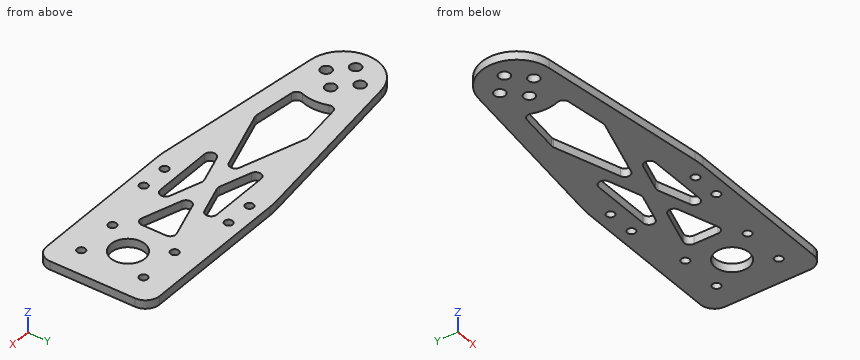
```python
from build123d import *

# Parameters (mm, degrees)
EXTRUDE_1_DEPTH          = 3
CUT_EXTRUDE_1_DEPTH      = 123.185310083
CUT_EXTRUDE_1_DEPTH_BACK = 123.185310083
SKETCH_2_R               = 1.95
FILLET_1_R               = 5
SKETCH_3_R               = 1.45
CUT_EXTRUDE_2_DEPTH      = 123.185310083
SKETCH_4_R               = 1.45
CUT_EXTRUDE_3_DEPTH      = 123.185310083
FILLET_2_R               = 30
SKETCH_6_R               = 6
CUT_EXTRUDE_4_DEPTH      = 123.185310083
FILLET_3_R               = 2


with BuildPart() as part:
    # 草图1 → 凸台-拉伸1 (new body)
    with BuildSketch(Plane.XY):
        with BuildLine():
            Line((60.5, 20), (120.5, 20))
            Line((120.5, 20), (120.5, -20))
            Line((120.5, -20), (60.5, -20))
            Line((60.5, -20), (-1.51896419, -12.407366674))
            ThreePointArc((-1.51896419, -12.407366674), (-12.5, 0), (-1.51896419, 12.407366674))
            Line((-1.51896419, 12.407366674), (60.5, 20))
        make_face()
    extrude(amount=EXTRUDE_1_DEPTH)

    # 草图2 → 切除-拉伸1 (cut, two sides: drawn at the far end of the back side and taken through both)
    with BuildSketch(Plane.XY.offset(3).offset(-CUT_EXTRUDE_1_DEPTH_BACK)):
        with Locations((0, 6)):
            Circle(SKETCH_2_R)
        with Locations((6, 0)):
            Circle(SKETCH_2_R)
        with Locations((0, -6)):
            Circle(SKETCH_2_R)
        with Locations((-6, 0)):
            Circle(SKETCH_2_R)
    extrude(amount=CUT_EXTRUDE_1_DEPTH + CUT_EXTRUDE_1_DEPTH_BACK, mode=Mode.SUBTRACT)

    # 圆角1
    fillet_1_edges = [part.edges().sort_by_distance(p)[0] for p in [
        (120.5, 20, 1.5),
        (120.5, -20, 1.5),
    ]]
    fillet(fillet_1_edges, radius=FILLET_1_R)

    # 草图3 → 切除-拉伸2 (cut, through all)
    with BuildSketch(Plane(origin=(0, 0, 0), x_dir=(-1, 0, 0), z_dir=(0, 0, -1))):
        with Locations((-111, -11)):
            Circle(SKETCH_3_R)
        with Locations((-111, 11)):
            Circle(SKETCH_3_R)
        with Locations((-96, 11)):
            Circle(SKETCH_3_R)
        with Locations((-96, -11)):
            Circle(SKETCH_3_R)
    extrude(amount=-CUT_EXTRUDE_2_DEPTH, mode=Mode.SUBTRACT)

    # 草图4 → 切除-拉伸3 (cut, through all)
    with BuildSketch(Plane.XY.offset(3)):
        with Locations((75.5, 15)):
            Circle(SKETCH_4_R)
        with Locations((65.5, 15)):
            Circle(SKETCH_4_R)
        with Locations(Location((65.5, -15, 0), (0, 0, 180))):
            Circle(SKETCH_4_R)
        with Locations(Location((75.5, -15, 0), (0, 0, 180))):
            Circle(SKETCH_4_R)
    extrude(amount=-CUT_EXTRUDE_3_DEPTH, mode=Mode.SUBTRACT)

    # 圆角2
    fillet_2_edges = [part.edges().sort_by_distance(p)[0] for p in [
        (60.5, 20, 1.5),
        (60.5, -20, 1.5),
    ]]
    fillet(fillet_2_edges, radius=FILLET_2_R)

    # 草图6 → 切除-拉伸4 (cut, through all)
    with BuildSketch(Plane.XY.offset(3)):
        with Locations((103.5, 0)):
            Circle(SKETCH_6_R)
        with BuildLine():
            Line((12.110641117, 7.023700714), (29.621886423, 9.167504088))
            Line((29.621886423, 9.167504088), (58.382978877, 0))
            Line((58.382978877, 0), (29.621886423, -9.167504088))
            Line((29.621886423, -9.167504088), (12.110641117, -7.023700714))
            ThreePointArc((12.110641117, -7.023700714), (14, 0), (12.110641117, 7.023700714))
        make_face()
        Polygon((40.181331173, -10), (63.710984536, -2.5), (87.240637899, -10), align=None)
        Polygon((40.181331173, 10), (63.710984536, 2.5), (87.240637899, 10), align=None)
        Polygon((91, 7), (69.038990194, 0), (91, -7), align=None)
    extrude(amount=-CUT_EXTRUDE_4_DEPTH, mode=Mode.SUBTRACT)

    # 圆角3
    fillet_3_edges = [part.edges().sort_by_distance(p)[0] for p in [
        (40.181331173, 10, 1.5),
        (87.240637899, 10, 1.5),
        (63.710984536, 2.5, 1.5),
        (91, 7, 1.5),
        (91, -7, 1.5),
        (69.038990194, 0, 1.5),
        (87.240637899, -10, 1.5),
        (40.181331173, -10, 1.5),
        (63.710984536, -2.5, 1.5),
        (12.110641117, -7.023700714, 1.5),
        (12.110641117, 7.023700714, 1.5),
        (29.621886423, 9.167504088, 1.5),
        (58.382978877, 0, 1.5),
        (29.621886423, -9.167504088, 1.5),
    ]]
    fillet(fillet_3_edges, radius=FILLET_3_R)


solid = part.part
```
Geometry check sheet. Reference: the model listing, model coordinates, mm. Round coordinates to 2 decimals unless told otherwise and drop trailing zeros. Order: outer loops, then holes, each group sorted by start corner. A loop starts at its lowest first (then second) coordinate and runs counter-clockwise, first axis right, second up. Notation, with made-up numbers: (57.5, -6.75) - (100.5, -6.75) arc R27 cw to (100.5, 19.25) - close; hole circle Ø7 at (10.25, 45). An arc over 180 degrees is marked (long way). Use a Markdown table: item, result. Add a question column.
(1) Sectioned sample at D-D, the plane x = 37. Enter the section's corners in (y, z).
(2) Material ranges on line 1 along Y through (x, z) = (111, 1.85); line 2 along Y through (x, z) = (71.5, 2.35); line 3 along Y through (x, z) = (103.5, 0.75), recorded low to high. Write a range as [from, to].
(3) Depth check by flat-ended pin: pin 1 (1 mm diameter, centred on y = 7.5, z = 0.5, fed in from -X). Enter the tip coordinate at first touch or a pass-through.
(4) Sectioned sample at B-B, the plane x = 65.5. Enter the section's corners in (y, z).
(5) Sectioned sample at A-A, the plane x = 103.5. Enter the section's corners in (y, z).
(6) Sectioned sample at C-C, the plane z = 0.85. Count the separate pieces of the cut face and the enclosed holes in it, and give its area (3 significant figures).
Answers below:
| question | item | result |
|---|---|---|
| 1 | outline | (-17.12, 0) - (-6.82, 0) - (-6.82, 3) - (-17.12, 3) - close; (6.82, 0) - (17.12, 0) - (17.12, 3) - (6.82, 3) - close |
| 2 | line 1 | [-20, -12.45], [-9.55, 9.55], [12.45, 20] |
| 2 | line 2 | [-20, -10], [-4.98, 4.98], [10, 20] |
| 2 | line 3 | [-20, -6], [6, 20] |
| 3 | pin 1 | x = -10.36 |
| 4 | outline | (-20, 0) - (-16.45, 0) - (-16.45, 3) - (-20, 3) - close; (-13.55, 0) - (-10, 0) - (-10, 3) - (-13.55, 3) - close; (-3.07, 0) - (3.07, 0) - (3.07, 3) - (-3.07, 3) - close; (10, 0) - (13.55, 0) - (13.55, 3) - (10, 3) - close; (16.45, 0) - (20, 0) - (20, 3) - (16.45, 3) - close |
| 5 | outline | (-20, 0) - (-6, 0) - (-6, 3) - (-20, 3) - close; (6, 0) - (20, 0) - (20, 3) - (6, 3) - close |
| 6 | separate pieces | 1 |
| 6 | enclosed holes | 17 |
| 6 | area | 3,460 mm² |
